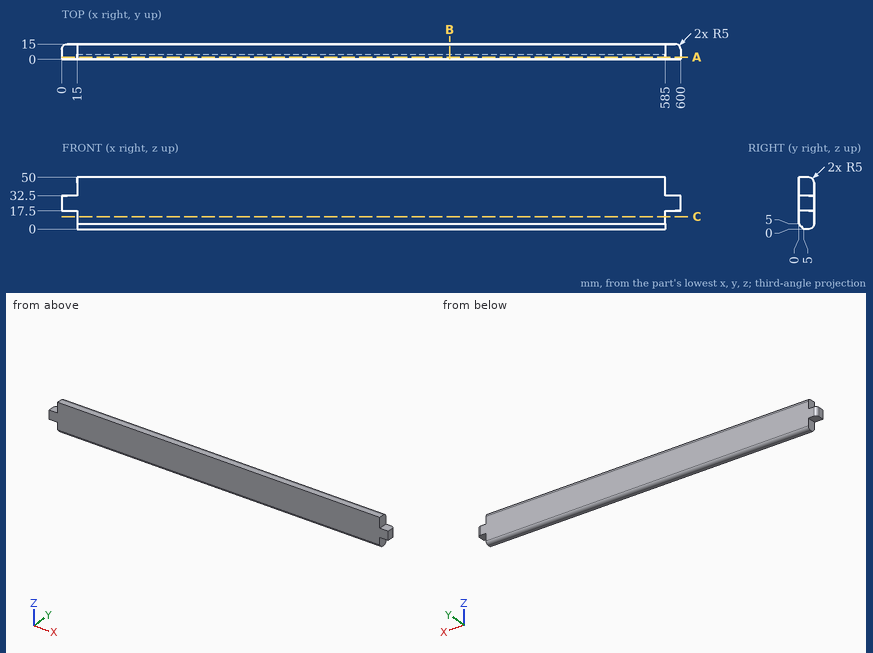
Here's the drawing with two shaded views (mm, measured from the low corner). I have some questions. Coordinates: 2 decimals unless noted, no trailing zeros. Write each loop counter-clockwise with the first axis right and the second up, starting at its lowest first coordinate (ties: lowest second). Pieces come first, ordered by that corner, then holes. Notation, with made-up numbers: (-33.75, 26.25) - (10.25, 26.25) arc R9 ccw to (10.25, 42.25) - close; hole circle Ø5 at (89.25, 15). An arc over 180 degrees is marked (long way). Return JSON: item names as keys, results as strings.
Q1. If we section it at C-C (z = 12): Please give me the cut outline in (x, y).
Computed values:
{"outline": "(15, 0) - (585, 0) - (585, 15) - (15, 15) - close"}
Q2. Please list where these lines run through material, in increasing order: L1, parallel to X at y = 11.25, z = 37.5; L2, parallel to Z at x = 404, y = 14; L3, parallel to Z at x = 530.5, y = 4.75. Write a range as from..to.
Computed values:
{"L1": "x = 15..585", "L2": "z = 2..48", "L3": "z = 0.25..50"}
Q3. If we section it at B-B (x = 376): Please give me the cut outline in (y, z), then the cut area to 3 significant figures.
Computed values:
{"outline": "(0, 5) - (5, 0) - (10, 0) arc R5 ccw to (15, 5) - (15, 45) arc R5 ccw to (10, 50) - (0, 50) - close", "area": "727 mm2"}
Q4. I'm going to push flat-ended pins straight in: pin 1 Ø4.5 at (x, y) = (7.5, 5) entering from +Z; pin 2 Ø4.5 at (y, z) = (5.5, 45) entering from -X; pin 3 Ø7.5 at (y, z) = (6, 39.5) entering from +X; pin 4 Ø5 at (y, z) = (2.5, 34) entering from +X. Where does each tip first touch, or does it pass through?
Computed values:
{"pin 1": "stops at z = 32.5", "pin 2": "stops at x = 15", "pin 3": "stops at x = 585", "pin 4": "stops at x = 600"}
Q5. If we section it at A-A (y = 2.25): Please give me the cut outline in (x, z).
Computed values:
{"outline": "(0, 17.5) - (15, 17.5) - (15, 2.75) - (585, 2.75) - (585, 17.5) - (600, 17.5) - (600, 32.5) - (585, 32.5) - (585, 50) - (15, 50) - (15, 32.5) - (0, 32.5) - close"}
